```python
from build123d import *

# Parameters (mm, degrees)
SKETCH1_W           = 56.891165124
SKETCH1_H           = 125.605714286
BOSS_EXTRUDE1_DEPTH = 2.54
CUT_EXTRUDE1_REACH  = 4.54
SKETCH2_R           = 12.7


with BuildPart() as part:
    # Sketch1 → Boss-Extrude1 (new body)
    with BuildSketch(Plane.XY):
        Rectangle(SKETCH1_W, SKETCH1_H)
    extrude(amount=BOSS_EXTRUDE1_DEPTH)

    # Sketch2 → Cut-Extrude1 (cut, up to next)
    with BuildSketch(Plane.XY.offset(2.54), mode=Mode.PRIVATE) as cut_extrude1_sk1:
        with Locations((0, 29.58)):
            Circle(SKETCH2_R)
    cut_extrude1_tool1 = extrude(cut_extrude1_sk1.sketch, amount=-CUT_EXTRUDE1_REACH, mode=Mode.PRIVATE) & part.part
    add(cut_extrude1_tool1.solids().sort_by_distance((0, 29.58, 2.54))[0], mode=Mode.SUBTRACT)
    # Sketch2 → Cut-Extrude1 (cut, up to next)
    with BuildSketch(Plane.XY.offset(2.54), mode=Mode.PRIVATE) as cut_extrude1_sk2:
        with Locations((0, -17.34)):
            Circle(SKETCH2_R)
    cut_extrude1_tool2 = extrude(cut_extrude1_sk2.sketch, amount=-CUT_EXTRUDE1_REACH, mode=Mode.PRIVATE) & part.part
    add(cut_extrude1_tool2.solids().sort_by_distance((0, -17.34, 2.54))[0], mode=Mode.SUBTRACT)


solid = part.part
```
Part model, mm, in its own coordinate system. Round coordinates to 2 decimals unless told otherwise and drop trailing zeros. Loops run counter-clockwise (first coordinate to the right, second up) from the corner with the lowest first, then second, coordinate; pieces in that order, holes last. Notation, with made-up numbers: (34.5, 73.5) -> (92.5, 73.5) arc R19 ccw to (92.5, 108.5) -> close; hole circle Ø8 at (-14.75, 72.5). An arc over 180 degrees is marked (long way). Use a Markdown table: item, result.
1) Probe line 1 (Y direction, x = 0, z = 0.65); line 2 (Y direction, x = 2, z = 0.2); line 3 (X direction, y = 27, z = 1.35). List the from-to ranges inside material, lowest first. Write a range as [from, to].
The answers:
| item | result |
|---|---|
| line 1 | y = [-62.8, -30.04], [-4.64, 16.88], [42.28, 62.8] |
| line 2 | y = [-62.8, -29.88], [-4.8, 17.04], [42.12, 62.8] |
| line 3 | x = [-28.45, -12.44], [12.44, 28.45] |
2) Drop a flat-ended pin along its axis: pin 1 Ø23 at (x, y) = (0, -17.34) entering from -Z. Give the stop position or say it passes through.
The answers:
| item | result |
|---|---|
| pin 1 | passes through |
3) Cut at B-B, the plane y = 29.58. List the corners of the cut face in (x, z), and give its area (3 significant figures).
The answers:
| item | result |
|---|---|
| outline | (-28.45, 0) -> (-12.7, 0) -> (-12.7, 2.54) -> (-28.45, 2.54) -> close; (12.7, 0) -> (28.45, 0) -> (28.45, 2.54) -> (12.7, 2.54) -> close |
| area | 80.0 mm2 |
4) Cut at A-A, the plane x = 0. List the corners of the cut face in (y, z), and give its area (3 significant figures).
The answers:
| item | result |
|---|---|
| outline | (-62.8, 0) -> (-30.04, 0) -> (-30.04, 2.54) -> (-62.8, 2.54) -> close; (-4.64, 0) -> (16.88, 0) -> (16.88, 2.54) -> (-4.64, 2.54) -> close; (42.28, 0) -> (62.8, 0) -> (62.8, 2.54) -> (42.28, 2.54) -> close |
| area | 190 mm2 |
5) Pull direction Y, two halves, no side cores. Call faces 1 (the flat face through (0, 62.803, 1)), 2 (the flat face through (0, 1, 0)), 3 (the cylindrical face through (-2.75, 17.18, 1.29)): pulls with the +Y half, pulls with the -Y half, needs draft (parallel to the pull), parting line crosses it, or undercut.
The answers:
| item | result |
|---|---|
| face 1 | pulls with the +Y half |
| face 2 | needs draft |
| face 3 | undercut |
6) Cut at C-C, the plane x = -7.5. List the corners of the cut face in (y, z).
The answers:
| item | result |
|---|---|
| outline | (-62.8, 0) -> (-27.59, 0) -> (-27.59, 2.54) -> (-62.8, 2.54) -> close; (-7.09, 0) -> (19.33, 0) -> (19.33, 2.54) -> (-7.09, 2.54) -> close; (39.83, 0) -> (62.8, 0) -> (62.8, 2.54) -> (39.83, 2.54) -> close |
